Geometry: final body of the model. Coordinates: model frame, mm. A direction names the side the tool comes from. Give positions to 0.01 mm unless a question says otherwise; leave off trailing zeros. Loops run counter-clockwise (first coordinate to the right, second up) from the corner with the lowest first, then second, coordinate; pieces in that order, holes last.
1. First-contact query: P1, Ø2.5, axis at y = 35.5, z = 3.5, coming from the -X side; P2, Ø1.5, axis at y = 21, z = 3, coming from the +X side. Flat tips, straight axial feed; report the tip coordinate or a pass-through.
2. Material intervals for line 1 along X through (y, z) = (-32, 0.3), sorted ascending.
3. Section B-B, the plane y = 15.5. Output: boundary loops of the cut face in (x, z).
4. Access query for faces 4 (the face through (88, 50, 3)), 5 (the face through (-90, 0, 2)), 6 (the face through (-88, 10, 3)). Directions: +Z, -Z, +X, -X, +Y, -Y. A direction counts if a zero-diameter tool reaches every point of the face in a straight line with its end or side. Return the directions, or none.
5. Section A-A, the plane z = 1.6. Output: boundary loops of the cut face in (x, y), then the cut area to 3 significant figures.
6. Draft query along Y for faces 1 (the face through (88, -50, 3)), 2 (the face through (90, 0, 2)), 3 (the face through (-1, -70, 2)). Return one class per face: +Y half, -Y half, draft (parallel to the pull), parting line (faces both ways), or undercut.
from build123d import *

# Parameters (mm, degrees)
CROQUIS1_W                = 180
CROQUIS1_H                = 140
SALIENTE_EXTRUIR1_DEPTH   = 5
CROQUIS4_W                = 5
CROQUIS4_H                = 40
CORTAR_EXTRUIR3_DEPTH     = 115.127122105
SIMETR_A5_COPY_1_SKETCH_W = 5
SIMETR_A5_COPY_1_SKETCH_H = 40
SIMETR_A5_COPY_1_DEPTH    = 115.127122105


with BuildPart() as part:
    # Croquis1 → Saliente-Extruir1 (new body)
    with BuildSketch(Plane.XY):
        Rectangle(CROQUIS1_W, CROQUIS1_H)
    extrude(amount=SALIENTE_EXTRUIR1_DEPTH)

    # Croquis4 → Cortar-Extruir3 (cut, through all)
    with BuildSketch(Plane.XY.offset(5)):
        with Locations((-87.5, 30)):
            Rectangle(CROQUIS4_W, CROQUIS4_H)
    cortar_extruir3 = extrude(amount=-CORTAR_EXTRUIR3_DEPTH, mode=Mode.SUBTRACT)

    # Simetría4: Cortar-Extruir3 across plane
    add(cortar_extruir3.mirror(Plane.ZX), mode=Mode.SUBTRACT)

    # Simetría5: Cortar-Extruir3 across plane
    add(cortar_extruir3.mirror(Plane(origin=(0, 0, 0), x_dir=(0, 0, 1), z_dir=(1, 0, 0))), mode=Mode.SUBTRACT)

    # Simetría5 copy 1 sketch → Simetría5 copy 1 (cut, through all)
    with BuildSketch(Plane(origin=(0, 0, 5), x_dir=(-1, 0, 0), z_dir=(0, 0, 1))):
        with Locations((-87.5, 30)):
            Rectangle(SIMETR_A5_COPY_1_SKETCH_W, SIMETR_A5_COPY_1_SKETCH_H)
    extrude(amount=-SIMETR_A5_COPY_1_DEPTH, mode=Mode.SUBTRACT)


solid = part.part
Answers below:
1. P1: stops at x = -85
1. P2: stops at x = 85
2. line 1: x = -85 to 85
3. outline: (-85, 0) - (85, 0) - (85, 5) - (-85, 5) - close
4. face 4: +Z, -Z, +X
4. face 5: +Z, -Z, -X, +Y, -Y
4. face 6: +Z, -Z, -X
5. outline: (-90, -70) - (90, -70) - (90, -50) - (85, -50) - (85, -10) - (90, -10) - (90, 10) - (85, 10) - (85, 50) - (90, 50) - (90, 70) - (-90, 70) - (-90, 50) - (-85, 50) - (-85, 10) - (-90, 10) - (-90, -10) - (-85, -10) - (-85, -50) - (-90, -50) - close
5. area: 24,400 mm2
6. face 1: undercut
6. face 2: draft
6. face 3: -Y half
